Model file for the job. Use its own axes, mm. Face numbers are marked on the shaded views. A direction names the side the tool comes from. Round coordinates to 2 decimals unless told otherwise and drop trailing zeros. Order: outer loops, then holes, each group sorted by start corner. A loop starts at its lowest first (then second) coordinate and runs counter-clockwise, first axis right, second up. Notation, with made-up numbers: (23.25, 55.5) -> (32.25, 55.5) arc R25 ccw to (32.25, 81.5) -> close; hole circle Ø11 at (-40, 3.5). An arc over 180 degrees is marked (long way). Answer as CSV lines item,"result".
```python
from build123d import *

# Parameters (mm, degrees)
BOSS_EXTRUDE1_DEPTH            = 15
F_2_CLEARANCE_HOLE1_AT_2_COUNT = 2
F_2_CLEARANCE_HOLE1_AT_2_PITCH = 6.096
F_6_START                      = 87.9325
F_6_CLEARANCE_HOLE1_OUTLINE_R  = 1.89865
F_6_CLEARANCE_HOLE1_DEPTH      = 1.5875
F_6_CLEARANCE_HOLE2_D          = 3.7973


# Read off the part's stored shape, not the designer's step: #6 Clearance Hole1
with BuildPart() as part:
    # Sketch1 → Boss-Extrude1 (new, symmetric)
    with BuildSketch(Plane.XY):
        Polygon((0, 0), (-65, 0), (-65, 89.52), (-25, 89.52), (-25, 87.9325), (-63.4125, 87.9325), (-63.4125, 1.5875), (0, 1.5875), align=None)
    boss_extrude1 = extrude(amount=BOSS_EXTRUDE1_DEPTH, both=True)

    # Sketch2 → #2 Clearance Hole1 (revolve, cut)
    with BuildSketch(Plane(origin=(-51.096, 0, 0), x_dir=(0, 0, -1), z_dir=(1, 0, 0))):
        Polygon((0, 0), (0, 2.252569267), (1.2192, 1.52), (1.2192, 0), align=None)
    f_2_clearance_hole1 = revolve(axis=Axis((-51.096, -6.35, 0), (0, 1, 0)), mode=Mode.SUBTRACT)

    # #2 Clearance Hole1 at 2: #2 Clearance Hole1 ×2
    with Locations(*[(i * F_2_CLEARANCE_HOLE1_AT_2_PITCH, 0, 0) for i in range(1, F_2_CLEARANCE_HOLE1_AT_2_COUNT)]):
        add(f_2_clearance_hole1, mode=Mode.SUBTRACT)

    # #6 Clearance Hole1 outline → #6 Clearance Hole1 (cut)
    with BuildSketch(Plane(origin=(0, 0, 0), x_dir=(1, 0, 0), z_dir=(0, 1, 0)).offset(F_6_START)):
        with Locations((-55, 0)):
            Circle(F_6_CLEARANCE_HOLE1_OUTLINE_R)
        with Locations((-35, 0)):
            Circle(F_6_CLEARANCE_HOLE1_OUTLINE_R)
    f_6_clearance_hole1 = extrude(amount=F_6_CLEARANCE_HOLE1_DEPTH, mode=Mode.SUBTRACT)

    # Mirror2: Boss-Extrude1, #2 Clearance Hole1, #6 Clearance Hole1 across plane
    add(boss_extrude1.mirror(Plane(origin=(0, 1.5875, -15), x_dir=(0, 0, 1), z_dir=(1, 0, 0))))
    add(f_2_clearance_hole1.mirror(Plane(origin=(0, 1.5875, -15), x_dir=(0, 0, 1), z_dir=(1, 0, 0))), mode=Mode.SUBTRACT)
    add(f_6_clearance_hole1.mirror(Plane(origin=(0, 1.5875, -15), x_dir=(0, 0, 1), z_dir=(1, 0, 0))), mode=Mode.SUBTRACT)

    # Mirror2 copy 1 sketch → Mirror2 copy 1 (revolve, cut)
    with BuildSketch(Plane(origin=(45, 0, 0), x_dir=(0, 0, -1), z_dir=(-1, 0, 0))):
        Polygon((0, 0), (0, -2.252569267), (1.2192, -1.52), (1.2192, 0), align=None)
    revolve(axis=Axis((45, -6.35, 0), (0, -1, 0)), mode=Mode.SUBTRACT)

    # #6 Clearance Hole2 (through all)
    with Locations(Plane(origin=(0, 0, 0), x_dir=(-1, 0, 0), z_dir=(0, -1, 0))):
        with Locations((-10, 0)):
            f_6_clearance_hole2 = Hole(F_6_CLEARANCE_HOLE2_D / 2)

    # Mirror3: #6 Clearance Hole2 across plane
    add(f_6_clearance_hole2.mirror(Plane(origin=(0, 0, 0), x_dir=(0, 0, 1), z_dir=(1, 0, 0))), mode=Mode.SUBTRACT)


solid = part.part
```
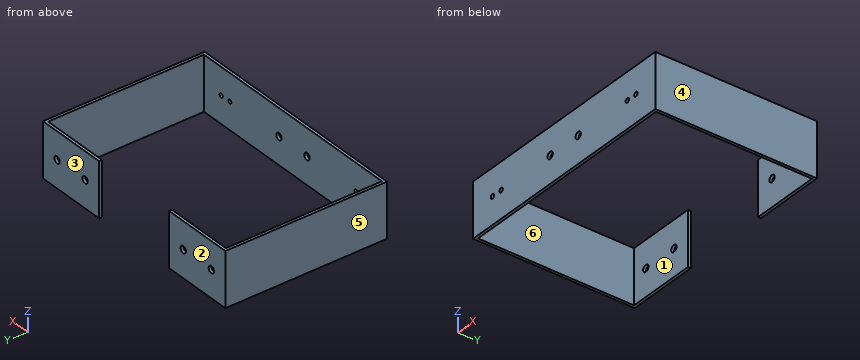
Q1. Saw through at B-B (x = -55). Write the cut outline in (y, z).
Checks:
outline,"(0, -15) -> (1.59, -15) -> (1.59, 15) -> (0, 15) -> close; (87.93, -15) -> (89.52, -15) -> (89.52, -1.9) -> (87.93, -1.9) -> close; (87.93, 1.9) -> (89.52, 1.9) -> (89.52, 15) -> (87.93, 15) -> close"
Q2. Saw through at D-D (z = -10.5). Write the cut outline in (x, y), plus the area to 3 significant figures.
Checks:
outline,"(-65, 0) -> (65, 0) -> (65, 89.52) -> (25, 89.52) -> (25, 87.93) -> (63.41, 87.93) -> (63.41, 1.59) -> (-63.41, 1.59) -> (-63.41, 87.93) -> (-25, 87.93) -> (-25, 89.52) -> (-65, 89.52) -> close"
area,"608 mm²"
Q3. Wall check: L1, parallel to X at y = 89, z = 0; L2, parallel to Z at x = 55, y = 88.3; L3, parallel to Y at x = -49, z = -10. Give the ranges that are in metal, low to high. Write a range as [from, to].
Checks:
L1,"[-65, -56.9], [-53.1, -36.9], [-33.1, -25], [25, 33.1], [36.9, 53.1], [56.9, 65]"
L2,"[-15, -1.9], [1.9, 15]"
L3,"[0, 1.59], [87.93, 89.52]"
Q4. Flat gauge pins, fed straight in: pin 1 (2 mm diameter, centred on x = -51.096, z = 0, fed in from -Y); pin 2 (9 mm diameter, centred on x = -18, z = -6, fed in from +Y). Where does each tip first touch, or does it go through?
Checks:
pin 1,"y = 87.93"
pin 2,"y = 1.59"
Q5. Saw through at A-A (x = -28). Write the cut outline in (y, z), plus the area to 4 significant figures.
Checks:
outline,"(0, -15) -> (1.59, -15) -> (1.59, 15) -> (0, 15) -> close; (87.93, -15) -> (89.52, -15) -> (89.52, 15) -> (87.93, 15) -> close"
area,"95.25 mm²"
Q6. Tool access for the marked faces 1 and 2: list every direction of +Z, -Z, +X, -X, +Y, -Y with a clear straight run to the whole face (end or side of a thin tool).
Checks:
face 1,"+Z, -Z"
face 2,"+Z, -Z, +X, -X, +Y"
Q7. Saw through at C-C (y = 58.5). Write the cut outline in (x, z).
Checks:
outline,"(-65, -15) -> (-63.41, -15) -> (-63.41, 15) -> (-65, 15) -> close; (63.41, -15) -> (65, -15) -> (65, 15) -> (63.41, 15) -> close"
Q8. Mould opens along X. For the marked faces 3, 4, 5 and 6 say: +X half, -X half, draft (parallel to the pull), parting line (faces both ways), or undercut.
Checks:
face 3,"draft"
face 4,"+X half"
face 5,"-X half"
face 6,"undercut"
